Design review of the part built by this model. Coordinates are the model's own, in mm. Give positions to 0.01 mm unless a question says otherwise; leave off trailing zeros. Write each loop counter-clockwise with the first axis right and the second up, starting at its lowest first coordinate (ties: lowest second). Pieces come first, ordered by that corner, then holes. Notation, with made-up numbers: (-12.5, -9) - (46.5, -9) arc R22 cw to (46.5, 4) - close; hole circle Ø11 at (42, 16.5). An arc over 180 degrees is marked (long way). Use a Markdown table: item, result. Add a question column.
```python
from build123d import *

# Parameters (mm, degrees)
SKETCH1_R           = 5
SKETCH1_R_2         = 3.7
BOSS_EXTRUDE1_DEPTH = 2
CHAMFER1_SIZE       = 0.3
CHAMFER2_SIZE       = 0.5


with BuildPart() as part:
    # Sketch1 → Boss-Extrude1 (new body)
    with BuildSketch(Plane.XY):
        Circle(SKETCH1_R)
        Circle(SKETCH1_R_2, mode=Mode.SUBTRACT)
    extrude(amount=BOSS_EXTRUDE1_DEPTH)

    # Chamfer1
    chamfer1_edges = [part.edges().sort_by_distance(p)[0] for p in [
        (-5, 0, 2),
    ]]
    chamfer(chamfer1_edges, length=CHAMFER1_SIZE)

    # Chamfer2
    chamfer2_edges = [part.edges().sort_by_distance(p)[0] for p in [
        (-3.7, 0, 0),
        (-3.7, 0, 2),
    ]]
    chamfer(chamfer2_edges, length=CHAMFER2_SIZE)


solid = part.part
```
(1) Add section A-A (y = 0). State the section outline as (x, z) points.
(2) Add section C-C (z = 0.9). State the section outline as (x, y) points, and give its area (3 significant figures).
(3) For line 1 along Y through (x, z) = (0, 0.95); line 2 along X through (y, z) = (-2, 1.2); line 3 along Y through (x, z) = (-3.5, 1.75), list the stretches that pass through material, from the lowest coordinate up.
(4) Mouldability with a two-part tool opening along X and no side actions: class faces 1 (the face through (-1.08, -4.88, 0.84)), 2 (the face through (-0.802, -3.612, 0.993)), 3 (the face through (-4, -2, 2)) as +X half, -X half, draft (parallel to the pull), parting line (faces both ways), or undercut.
Answers follow:
| question | item | result |
|---|---|---|
| 1 | outline | (-5, 0) - (-4.2, 0) - (-3.7, 0.5) - (-3.7, 1.5) - (-4.2, 2) - (-4.7, 2) - (-5, 1.7) - close; (3.7, 0.5) - (4.2, 0) - (5, 0) - (5, 1.7) - (4.7, 2) - (4.2, 2) - (3.7, 1.5) - close |
| 2 | outline | circle Ø10 at (0, 0); hole circle Ø7.4 at (0, 0) |
| 2 | area | 35.5 mm^2 |
| 3 | line 1 | -5 to -3.7, 3.7 to 5 |
| 3 | line 2 | -4.58 to -3.11, 3.11 to 4.58 |
| 3 | line 3 | -3.5 to -1.83, 1.83 to 3.5 |
| 4 | face 1 | parting line |
| 4 | face 2 | undercut |
| 4 | face 3 | draft |
